Design review of the part built by this model. Coordinates are the model's own, in mm. Face numbers are marked on the shaded views. A direction names the side the tool comes from. Coordinates: 2 decimals unless noted, no trailing zeros. Write each loop counter-clockwise with the first axis right and the second up, starting at its lowest first coordinate (ties: lowest second). Pieces come first, ordered by that corner, then holes. Notation, with made-up numbers: (65, 70) - (92, 70) arc R21 cw to (92, 83) - close; hole circle Ø4 at (6.25, 23.25). An arc over 180 degrees is marked (long way). Use a Markdown table: item, result.
from build123d import *

# Parameters (mm, degrees)
F0_R     = 3.175
F0_R_2   = 3.9751
F1_DEPTH = 3.175
F2_DEPTH = 3.175


# Not quite as in the source:
# - after a boolean that leaves OpenCascade's solid faulty, fix() repairs it


with BuildPart() as f1:
    # F0 (on Top) → F1 (new body)
    with BuildSketch(Plane.XY):
        with BuildLine():
            Line((0.1954344954, -20.7710836138), (-10.1235074968, -12.2282550252))
            ThreePointArc((-10.1235074968, -12.2282550252), (-11.1192092809, -11.3304373246), (-12.0356034274, -10.3518054047))
            Line((-12.0356034274, -10.3518054047), (-20.9391765456, 0))
            Line((-20.9391765456, 0), (-42.5571087943, -25.134249466))
            ThreePointArc((-42.5571087943, -25.134249466), (-47.4235249822, -27.815033629), (-52.8569612369, -26.6546971654))
            Line((-52.8569612369, -26.6546971654), (-76.3196547531, -11.7034610596))
            ThreePointArc((-76.3196547531, -11.7034610596), (-73.6260110422, -14.5799404883), (-72.6477527528, -18.3973821792))
            ThreePointArc((-72.6477527528, -18.3973821792), (-77.2746501981, -25.611522251), (-85.7611554551, -24.4151838929))
            Line((-85.7611554551, -24.4151838929), (-52.1475443887, -53.3262030046))
            ThreePointArc((-52.1475443887, -53.3262030046), (-49.5361241819, -34.8014845049), (-33.7887806053, -44.9012806053))
            ThreePointArc((-33.7887806053, -44.9012806053), (-34.8014845049, -49.5361241819), (-37.655016822, -53.3262030046))
            Line((-37.655016822, -53.3262030046), (0.1954344954, -20.7710836138))
        make_face()
        with Locations((-30.2993841525, -30.2993841525)):
            Circle(F0_R, mode=Mode.SUBTRACT)
        with BuildLine():
            ThreePointArc((-52.1475443887, -53.3262030046), (-44.9012806053, -56.0137806053), (-37.655016822, -53.3262030046))
            ThreePointArc((-37.655016822, -53.3262030046), (-34.8014845049, -49.5361241819), (-33.7887806053, -44.9012806053))
            ThreePointArc((-33.7887806053, -44.9012806053), (-49.5361241819, -34.8014845049), (-52.1475443887, -53.3262030046))
        make_face()
        with BuildLine():
            ThreePointArc((-76.3196547531, -11.7034610596), (-86.9573903855, -13.664542837), (-85.7611554551, -24.4151838929))
            ThreePointArc((-85.7611554551, -24.4151838929), (-77.2746501981, -25.611522251), (-72.6477527528, -18.3973821792))
            ThreePointArc((-72.6477527528, -18.3973821792), (-73.6260110422, -14.5799404883), (-76.3196547531, -11.7034610596))
        make_face()
        with Locations((-80.5852527528, -18.3973821792)):
            Circle(F0_R, mode=Mode.SUBTRACT)
        with BuildLine():
            Line((0.1954344954, -20.7710836138), (10.3518055249, -12.0356033241))
            ThreePointArc((10.3518055249, -12.0356033241), (0.1493608613, -15.8742973493), (-10.1235074968, -12.2282550252))
            Line((-10.1235074968, -12.2282550252), (0.1954344954, -20.7710836138))
        make_face()
        with BuildLine():
            ThreePointArc((-12.0356034274, -10.3518054047), (-15.875, 6.76e-08), (-12.0356033393, 10.3518055072))
            Line((-12.0356033393, 10.3518055072), (-20.9391765456, 0))
            Line((-20.9391765456, 0), (-12.0356034274, -10.3518054047))
        make_face()
        with BuildLine():
            ThreePointArc((10.3518055249, -12.0356033241), (14.4282801766, -6.6212050373), (15.875, 0))
            ThreePointArc((15.875, 0), (14.9355142785, 5.3801522504), (12.2282550252, 10.1235074968))
            ThreePointArc((12.2282550252, 10.1235074968), (11.3304373246, 11.1192092809), (10.3518054047, 12.0356034274))
            ThreePointArc((10.3518054047, 12.0356034274), (-1.1906249326, 15.8302886035), (-12.0356033393, 10.3518055072))
            ThreePointArc((-12.0356033393, 10.3518055072), (-15.875, 6.76e-08), (-12.0356034274, -10.3518054047))
            ThreePointArc((-12.0356034274, -10.3518054047), (-11.1192092809, -11.3304373246), (-10.1235074968, -12.2282550252))
            ThreePointArc((-10.1235074968, -12.2282550252), (0.1493608613, -15.8742973493), (10.3518055249, -12.0356033241))
        make_face()
        Circle(F0_R_2, mode=Mode.SUBTRACT)
    extrude(amount=-F1_DEPTH)

    # F0 (on Top) → F2 (join)
    with BuildSketch(Plane.XY):
        with BuildLine():
            ThreePointArc((-12.0356033393, 10.3518055072), (-1.1906249326, 15.8302886035), (10.3518054047, 12.0356034274))
            Line((10.3518054047, 12.0356034274), (-37.655016822, 53.3262030046))
            ThreePointArc((-37.655016822, 53.3262030046), (-34.8014845049, 49.5361241819), (-33.7887806053, 44.9012806053))
            ThreePointArc((-33.7887806053, 44.9012806053), (-49.5361241819, 34.8014845049), (-52.1475443887, 53.3262030046))
            Line((-52.1475443887, 53.3262030046), (-85.7611554551, 24.4151838929))
            ThreePointArc((-85.7611554551, 24.4151838929), (-77.2746501981, 25.611522251), (-72.6477527528, 18.3973821792))
            ThreePointArc((-72.6477527528, 18.3973821792), (-73.6260112444, 14.5799401196), (-76.3196554623, 11.7034606077))
            Line((-76.3196554623, 11.7034606077), (-52.8569612369, 26.6546971654))
            ThreePointArc((-52.8569612369, 26.6546971654), (-47.4235249822, 27.815033629), (-42.5571087943, 25.134249466))
            Line((-42.5571087943, 25.134249466), (-20.9391765456, 0))
            Line((-20.9391765456, 0), (-12.0356033393, 10.3518055072))
        make_face()
        with BuildLine():
            ThreePointArc((-72.6477527528, 18.3973821792), (-77.2746501981, 25.611522251), (-85.7611554551, 24.4151838929))
            ThreePointArc((-85.7611554551, 24.4151838929), (-86.9573906362, 13.6645431745), (-76.3196554623, 11.7034606077))
            ThreePointArc((-76.3196554623, 11.7034606077), (-73.6260112444, 14.5799401196), (-72.6477527528, 18.3973821792))
        make_face()
        with Locations((-80.5852527528, 18.3973821792)):
            Circle(F0_R, mode=Mode.SUBTRACT)
        with BuildLine():
            ThreePointArc((-33.7887806053, 44.9012806053), (-34.8014845049, 49.5361241819), (-37.655016822, 53.3262030046))
            ThreePointArc((-37.655016822, 53.3262030046), (-44.9012806053, 56.0137806053), (-52.1475443887, 53.3262030046))
            ThreePointArc((-52.1475443887, 53.3262030046), (-49.5361241819, 34.8014845049), (-33.7887806053, 44.9012806053))
        make_face()
        with Locations((-44.9012806053, 44.9012806053)):
            Circle(F0_R, mode=Mode.SUBTRACT)
        with BuildLine():
            ThreePointArc((10.3518055249, -12.0356033241), (14.4282801766, -6.6212050373), (15.875, 0))
            ThreePointArc((15.875, 0), (14.9355142785, 5.3801522504), (12.2282550252, 10.1235074968))
            ThreePointArc((12.2282550252, 10.1235074968), (11.3304373246, 11.1192092809), (10.3518054047, 12.0356034274))
            ThreePointArc((10.3518054047, 12.0356034274), (-1.1906249326, 15.8302886035), (-12.0356033393, 10.3518055072))
            ThreePointArc((-12.0356033393, 10.3518055072), (-15.875, 6.76e-08), (-12.0356034274, -10.3518054047))
            ThreePointArc((-12.0356034274, -10.3518054047), (-11.1192092809, -11.3304373246), (-10.1235074968, -12.2282550252))
            ThreePointArc((-10.1235074968, -12.2282550252), (0.1493608613, -15.8742973493), (10.3518055249, -12.0356033241))
        make_face()
        Circle(F0_R_2, mode=Mode.SUBTRACT)
        with BuildLine():
            ThreePointArc((-12.0356034274, -10.3518054047), (-15.875, 6.76e-08), (-12.0356033393, 10.3518055072))
            Line((-12.0356033393, 10.3518055072), (-20.9391765456, 0))
            Line((-20.9391765456, 0), (-12.0356034274, -10.3518054047))
        make_face()
        with BuildLine():
            Line((0.1954344954, -20.7710836138), (10.3518055249, -12.0356033241))
            ThreePointArc((10.3518055249, -12.0356033241), (0.1493608613, -15.8742973493), (-10.1235074968, -12.2282550252))
            Line((-10.1235074968, -12.2282550252), (0.1954344954, -20.7710836138))
        make_face()
        with BuildLine():
            ThreePointArc((12.2282550252, 10.1235074968), (14.9355142785, 5.3801522504), (15.875, 0))
            ThreePointArc((15.875, 0), (14.4282801766, -6.6212050373), (10.3518055249, -12.0356033241))
            Line((10.3518055249, -12.0356033241), (0.1954344954, -20.7710836138))
            Line((0.1954344954, -20.7710836138), (28.8345692365, -44.4808030019))
            ThreePointArc((28.8345692365, -44.4808030019), (24.8320655021, -35.1980826181), (30.0059355892, -26.5136135964))
            ThreePointArc((30.0059355892, -26.5136135964), (37.6803722933, -24.9486796329), (44.4808030542, -28.8345692997))
            Line((44.4808030542, -28.8345692997), (12.2282550252, 10.1235074968))
        make_face()
        with BuildLine():
            ThreePointArc((31.490910058, -23.8257819975), (31.094979692, -25.361163699), (30.0059355892, -26.5136135964))
            ThreePointArc((30.0059355892, -26.5136135964), (25.536840424, -22.290400296), (31.490910058, -23.8257819975))
        make_face(mode=Mode.SUBTRACT)
        with BuildLine():
            ThreePointArc((47.0335244843, -35.9210244843), (46.3758844931, -32.1549179476), (44.4808030542, -28.8345692997))
            ThreePointArc((44.4808030542, -28.8345692997), (37.6803722933, -24.9486796329), (30.0059355892, -26.5136135964))
            ThreePointArc((30.0059355892, -26.5136135964), (24.8320655021, -35.1980826181), (28.8345692365, -44.4808030019))
            ThreePointArc((28.8345692365, -44.4808030019), (40.650687385, -45.9767663811), (47.0335244843, -35.9210244843))
        make_face()
        with Locations((35.9210244843, -35.9210244843)):
            Circle(F0_R, mode=Mode.SUBTRACT)
    extrude(amount=F2_DEPTH)

    add(f1.part.fix(), mode=Mode.REPLACE)


solid = f1.part
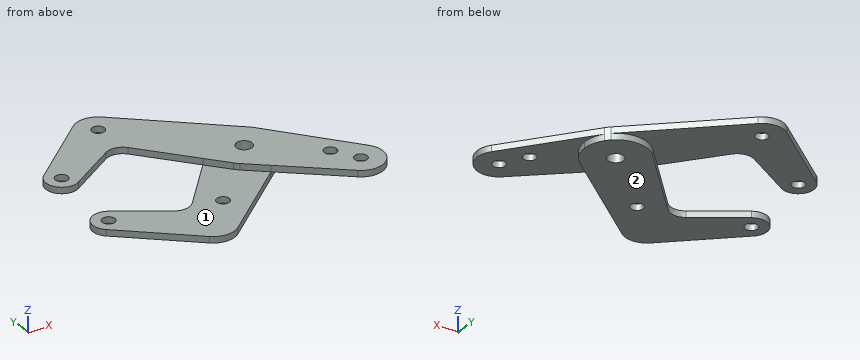
(1) Machinability: for the marked faces 1 and 2, which of the approach directions +Z, -Z, +X, -X, +Y, -Y give a long, thin tool a straight path to every point of the face, cutting with its end or side? Answer none if there is none.
Determined:
| item | result |
|---|---|
| face 1 | +Z, -X, -Y |
| face 2 | -Z, +X, -X, +Y, -Y |
(2) Take a section at B-B on y = -5.5. Write out the cut boundary in (x, z) (3 decimals), and give its area (3 significant figures).
Determined:
| item | result |
|---|---|
| outline | (-25.67, -3.175) - (14.892, -3.175) - (14.892, 0) - (25.163, 0) - (25.163, 3.175) - (-16.209, 3.175) - (-16.209, 0) - (-25.67, 0) - close |
| area | 260 mm2 |
(3) For L1, parallel to Z at x = -54, y = -36 (3 decimals); L2, parallel to Z at x = 35, y = -39 (3 decimals); L3, parallel to Y at x = -79, z = 2.75, list the stretches that pass through material, from the lowest coordinate up. Write a range as from..to.
Determined:
| item | result |
|---|---|
| L1 | -3.175..0 |
| L2 | 0..3.175 |
| L3 | 10.62..15.65, 21.15..30.23 |
(4) Take a section at A-A on y = 23. Write out the cut boundary in (x, z) (3 decimals), and give its area (3 significant figures).
Determined:
| item | result |
|---|---|
| outline | (-87.052, 0) - (-58.592, 0) - (-58.592, 3.175) - (-87.052, 3.175) - close; (-40.721, 0) - (-2.396, 0) - (-2.396, 3.175) - (-40.721, 3.175) - close |
| area | 212 mm2 |
(5) For pin 1 (10 mm diameter, centred on x = 28.32, y = -23.83, fed in from -Z); pin 2 (3 mm diameter, centred on y = 2, z = -1, fed in from +X); pin 3 (1.5 mm diameter, centred on y = -38.5, z = 0.5, fed in from -X), all flat-tipped, find the tip position at first contact; note any pin that passes through.
Determined:
| item | result |
|---|---|
| pin 1 | z = 0 |
| pin 2 | x = 19.88 |
| pin 3 | x = -70.04 |
